```python
from build123d import *

# Parameters (mm, degrees)
SKETCH1_R           = 21.5
BOSS_EXTRUDE1_DEPTH = 27
SKETCH2_R           = 18.75
CUT_EXTRUDE2_DEPTH  = 24
SKETCH4_W           = 3.3
SKETCH4_H           = 14
CUT_EXTRUDE6_DEPTH  = 32
SKETCH7_R           = 5
CUT_EXTRUDE8_DEPTH  = 1


with BuildPart() as part:
    # Sketch1 → Boss-Extrude1 (new body)
    with BuildSketch(Plane.XY):
        Circle(SKETCH1_R)
    extrude(amount=BOSS_EXTRUDE1_DEPTH)

    # Sketch2 → Cut-Extrude2 (cut)
    with BuildSketch(Plane.XY):
        Circle(SKETCH2_R)
    extrude(amount=CUT_EXTRUDE2_DEPTH, mode=Mode.SUBTRACT)

    # Sketch4 → Cut-Extrude6 (cut)
    with BuildSketch(Plane.XY):
        with Locations((13.8, 0)):
            Rectangle(SKETCH4_W, SKETCH4_H)
        with Locations((-13.8, 0)):
            Rectangle(SKETCH4_W, SKETCH4_H)
    extrude(amount=CUT_EXTRUDE6_DEPTH, mode=Mode.SUBTRACT)

    # Sketch7 → Cut-Extrude8 (cut)
    with BuildSketch(Plane.XY.offset(27)):
        Circle(SKETCH7_R)
    extrude(amount=-CUT_EXTRUDE8_DEPTH, mode=Mode.SUBTRACT)


solid = part.part
```
Read the model definition and answer for the solid it produces. Units are mm, in the model's axes. A direction names the side the tool comes from. Coordinates: 2 decimals unless noted, no trailing zeros. Write each loop counter-clockwise with the first axis right and the second up, starting at its lowest first coordinate (ties: lowest second). Pieces come first, ordered by that corner, then holes. Notation, with made-up numbers: (70.25, -32.5) -> (90.25, -32.5) arc R14 cw to (90.25, -15.5) -> close; hole circle Ø7 at (79.25, 18). An arc over 180 degrees is marked (long way). Write item = value, one per line.
(1) Which of the six approach directions +Z, -Z, +X, -X, +Y, -Y give full straight-line access (tool end or side, diameter ignored) to faces 5 (the face through (0, 0, 24)), 6 (the face through (-14, -7, 25)), 7 (the face through (0, 0, 26)), 8 (the face through (-6, 18, 0))?
From the geometry:
face_5 = -Z
face_6 = +Z, -Z
face_7 = +Z
face_8 = -Z, +X, -X, +Y, -Y
(2) Straight lines are drawn through the part: L1, parallel to Y at x = 0, z = 26.45; L2, parallel to Y at x = 0, z = 7.5; L3, parallel to Z at x = -7, y = -8.5. For each, find the intervals that lie inside material, in ascending order. Write a range as from..to.
From the geometry:
L1 = -21.5..-5, 5..21.5
L2 = -21.5..-18.75, 18.75..21.5
L3 = 24..27
(3) Given pin 1 Ø1 at (y, z) = (-11.5, 15) entering from +X; pin 2 Ø3.5 at (x, z) = (-13, 25) entering from +Y; pin 3 Ø0.9 at (x, z) = (14, 26) entering from +Y, each flat-ended and moving along its own axis, determine where each tip first touches the part or whether it passes through.
From the geometry:
pin_1 = 18.47
pin_2 = 18.32
pin_3 = 16.69
(4) Section A-A on y = 0 is taken. Write down the section's boundary in (x, z).
From the geometry:
outline = (-21.5, 0) -> (-18.75, 0) -> (-18.75, 24) -> (-15.45, 24) -> (-15.45, 27) -> (-21.5, 27) -> close; (-12.15, 24) -> (12.15, 24) -> (12.15, 27) -> (5, 27) -> (5, 26) -> (-5, 26) -> (-5, 27) -> (-12.15, 27) -> close; (15.45, 24) -> (18.75, 24) -> (18.75, 0) -> (21.5, 0) -> (21.5, 27) -> (15.45, 27) -> close
(5) For a pull along X with two mould halves and no side action, classify faces 1 (the face through (-14, 7, 25)), 2 (the face through (-2.799, 21.317, 13.311)), 3 (the face through (4, -4, 27)), 4 (the face through (-1.08, -4.88, 26.51)) as +X half, -X half, draft (parallel to the pull), parting line (faces both ways), or undercut.
From the geometry:
face_1 = undercut
face_2 = parting line
face_3 = draft
face_4 = undercut
(6) Section B-B on x = 0 is taken. Write down the section's boundary in (y, z), plus the area to 3 significant figures.
From the geometry:
outline = (-21.5, 0) -> (-18.75, 0) -> (-18.75, 24) -> (18.75, 24) -> (18.75, 0) -> (21.5, 0) -> (21.5, 27) -> (5, 27) -> (5, 26) -> (-5, 26) -> (-5, 27) -> (-21.5, 27) -> close
area = 251 mm2
(7) Section C-C on z = 17.5 is taken. Write down the section's boundary in (x, y), plus the area to 3 significant figures.
From the geometry:
outline = circle Ø43 at (0, 0); hole circle Ø37.5 at (0, 0)
area = 348 mm2
(8) Section D-D on x = -7 is taken. Write down the section's boundary in (y, z).
From the geometry:
outline = (-20.33, 0) -> (-17.39, 0) -> (-17.39, 24) -> (17.39, 24) -> (17.39, 0) -> (20.33, 0) -> (20.33, 27) -> (-20.33, 27) -> close
